Could you check a few things on this model? Use its own coordinates, in mm. A direction names the side the tool comes from. Coordinates: 2 decimals unless noted, no trailing zeros. Loops run counter-clockwise (first coordinate to the right, second up) from the corner with the lowest first, then second, coordinate; pieces in that order, holes last.
1) Will these pins go through, and if not, where does the flat tip stop? P1, Ø1.8, axis at x = -14, z = 15.5, coming from the -Y side; P2, Ø1.9, axis at x = 20, z = -37.5, coming from the -Y side; P3, Ø1.5, axis at x = -13, z = -19, coming from the +Y side; P4, Ø3, axis at x = 15.25, z = -15.25, coming from the +Y side.
2) Imagine slicing it at A-A on y = 11.25. Please give me the cut outline in (x, z).
3) For faces 3 (the face through (-15, 2.3, -15)), 4 (the face through (-21.31, 2.46, -36.67)), 5 (the face through (12.869, 11.451, 13.425)), which set-ups out of +Z, -Z, +X, -X, +Y, -Y let a thin tool reach every point of the face, with its end or its side?
4) Thinking about a two-plate mould opening in Z: for faces 1 (the face through (-12.869, 11.451, 17.075)), 2 (the face through (22.5, 2, -1)), which applies, released by +Z, released by -Z, zero draft, split by the parting line, or undercut?
5) Imagine slicing it at C-C on y = 1. Give the number of separate pieces and of enclosed holes in the cut face, plus the area to 3 significant figures.
6) Imagine slicing it at B-B on z = 37.5. Please give me the cut outline in (x, y), plus the area to 3 significant figures.
7) Imagine slicing it at D-D on x = 1. Please give me the cut outline in (y, z).
8) If I drill on line 1 along X through (y, z) = (1.05, 15.25); line 2 along Z through (x, y) = (15.25, 1.6); line 3 along Z through (x, y) = (-16.5, 9.5), over which ranges is the centre line in solid material (lowest first)?
Autodesk Inventor part; units mm, degrees
ref_plane "YZ Plane" through (0, 0, 0) normal (1, 0, 0) x (0, 1, 0)
ref_plane "XZ Plane" through (0, 0, 0) normal (0, 1, 0) x (-1, 0, 0)
ref_plane "XY Plane" through (0, 0, 0) normal (0, 0, 1) x (1, 0, 0)
sketch "Sketch1" plane through (0, 0, 0) normal (0, 1, 0) x (-1, 0, 0)
  line L0 (-22.5, 40) -> (22.5, 40)
  line L1 (22.5, 40) -> (22.5, -40)
  line L2 (22.5, -40) -> (-22.5, -40)
  line L3 (-22.5, -40) -> (-22.5, 40)
  line L4 (-22.5, 40) -> (22.5, -40) construction
  line L5 (22.5, 40) -> (-22.5, -40) construction
  point P0 (0, 0)
  dimension "d0" = 80
  dimension "d1" = 45
extrude "Extrusion1" add sketch "Sketch1" along normal blind 5
ref_plane "Work Plane1" through (22.5, 0, 0) normal (0, 0, -1) x (-1, 0, 0)
ref_plane "Work Plane2" through (0, 0, 40) normal (1, 0, 0) x (0, 0, -1)
sketch "Sketch2" plane through (0, 5, 0) normal (0, 1, 0) x (1, 0, 0)
  line L0 (-22.5, 40) -> (22.5, 40)
  line L1 (22.5, -40) -> (22.5, 40)
  point P0 (0, 0)
  point P1 (20, 37.5)
  dimension "d4" = 2.5
  dimension "d5" = 2.5
hole "Hole1" at (20, 5, -37.5) direction (0, -1, 0) diameter 3.1 end through all
fillet "Fillet1" radius 1 1 edges at (22.5, 2.5, -40)
sketch "Sketch3" plane through (0, 5, 0) normal (0, 1, 0) x (1, 0, 0)
  circle A0 centre (15.25, 15.25) radius 3
  line L0 (-31.5, 0) -> (31.5, 0) construction
  line L1 (0, 56) -> (0, -56) construction
  point P0 (0, 0)
  dimension "d14" = 15.25
  dimension "d15" = 15.25
  dimension "d16" = 6
extrude "Extrusion2" add sketch "Sketch3" along normal blind 10
hole "Hole2" at (15.25, 15, -15.25) direction (0, -1, 0) diameter 3.1 depth 11 tip angle 118
sketch "Sketch5" plane through (0, 0, 0) normal (0, -1, 0) x (1, 0, 0)
  circle A0 centre (15.25, -15.25) radius 3
  point P0 (0, 0)
extrude "Extrusion3" cut sketch "Sketch5" against normal blind 2.3
fillet "Fillet2" radius 3 1 edges at (12.25, 5, -15.25)
mirror "Mirror1" about plane through (0, 0, 40) normal (1, 0, 0) of "Hole2", "Extrusion2", "Fillet1", "Hole1", "Extrusion3", "Fillet2"
mirror "Mirror2" about plane through (22.5, 0, 0) normal (0, 0, -1) of "Hole2", "Extrusion2", "Fillet1", "Hole1", "Mirror1", "Extrusion3", "Fillet2"
sketch "Sketch4" plane through (0, 5, 0) normal (0, 1, 0) x (1, 0, 0)
  circle A0 centre (-20, -37.5) radius 1.55 construction
  line L0 (-21.5, -40) -> (21.5, -40) construction
  point P0 (0, 0)
  point P1 (10, -37.5)
  dimension "d30" = 30
hole "Hole3" at (10, 5, 37.5) direction (0, -1, 0) diameter 2 end through all
equation "\"d14\" = d15"
properties part number "porte_carte"
Filled in:
1. P1: stops at y = 2.3
1. P2: passes through
1. P3: stops at y = 6.17
1. P4: stops at y = 3.97
2. outline: circle Ø6 at (-15.25, -15.25); circle Ø6 at (-15.25, 15.25); circle Ø6 at (15.25, -15.25); circle Ø6 at (15.25, 15.25); hole circle Ø3.1 at (-15.25, -15.25); hole circle Ø3.1 at (-15.25, 15.25); hole circle Ø3.1 at (15.25, -15.25); hole circle Ø3.1 at (15.25, 15.25)
3. face 3: -Y
3. face 4: +Y, -Y
3. face 5: +Y
4. face 1: undercut
4. face 2: zero draft
5. separate pieces: 1
5. enclosed holes: 9
5. area: 3,450 mm2
6. outline: (-22.5, 0) - (-21.55, 0) - (-21.55, 5) - (-22.5, 5) - close; (-18.45, 0) - (9, 0) - (9, 5) - (-18.45, 5) - close; (11, 0) - (18.45, 0) - (18.45, 5) - (11, 5) - close; (21.55, 0) - (22.5, 0) - (22.5, 5) - (21.55, 5) - close
6. area: 184 mm2
7. outline: (0, -40) - (5, -40) - (5, 40) - (0, 40) - close
8. line 1: x = -22.5 to -18.25, -12.25 to 12.25, 18.25 to 22.5
8. line 2: z = -40 to -18.25, -12.25 to 12.25, 18.25 to 40
8. line 3: z = -17.98 to -16.17, -14.33 to -12.52, 12.52 to 14.33, 16.17 to 17.98
